from build123d import *

# Parameters (mm, degrees)
F0_R     = 26
F0_R_2   = 22.5
F0_R_3   = 15.5
F0_R_4   = 12.5
F1_DEPTH = 15
F3_R     = 5
F4_DEPTH = 11


with BuildPart() as f1:
    # F0 (on Front) → F1 (new body)
    with BuildSketch(Plane.XZ):
        Circle(F0_R)
        Circle(F0_R_2, mode=Mode.SUBTRACT)
        Circle(F0_R_3)
        Circle(F0_R_4, mode=Mode.SUBTRACT)
    extrude(amount=F1_DEPTH)

    # F3 (on offset) → F4 (join)
    with BuildSketch(Plane.XZ.offset(2)):
        with Locations((0, 19)):
            Circle(F3_R)
        with Locations((11.16792, 15.371323)):
            Circle(F3_R)
        with Locations((18.070074, 5.871323)):
            Circle(F3_R)
        with Locations((18.070074, -5.871323)):
            Circle(F3_R)
        with Locations((11.16792, -15.371323)):
            Circle(F3_R)
        with Locations((0, -19)):
            Circle(F3_R)
        with Locations((-11.16792, -15.371323)):
            Circle(F3_R)
        with Locations((-18.070074, -5.871323)):
            Circle(F3_R)
        with Locations((-18.070074, 5.871323)):
            Circle(F3_R)
        with Locations((-11.16792, 15.371323)):
            Circle(F3_R)
    extrude(amount=F4_DEPTH)


solid = f1.part
Build history of the part. All positions in model axes, mm. A direction names the side the tool comes from. Round coordinates to 2 decimals unless told otherwise and drop trailing zeros. Write each loop counter-clockwise with the first axis right and the second up, starting at its lowest first coordinate (ties: lowest second). Pieces come first, ordered by that corner, then holes. Notation, with made-up numbers: M 2.25,32 L 22.25,32 A26 cw 22.25,60 Z; hole C 68.5,-13 d6. An arc over 180 degrees is marked long. Answer in a Markdown table with one row per item.
1. Saw through at A-A (x = 0). List the corners of the cut face in (y, z), and give its area (3 significant figures).
Geometry check:
| item | result |
|---|---|
| outline | M -15,-26 L 0,-26 L 0,-22.5 L -2,-22.5 L -2,-15.5 L 0,-15.5 L 0,-12.5 L -15,-12.5 L -15,-15.5 L -13,-15.5 L -13,-22.5 L -15,-22.5 Z; M -15,12.5 L 0,12.5 L 0,15.5 L -2,15.5 L -2,22.5 L 0,22.5 L 0,26 L -15,26 L -15,22.5 L -13,22.5 L -13,15.5 L -15,15.5 Z |
| area | 349 mm2 |
2. Mould opens along Z. For faces 1 (the face through (-16.033, -7.423, 10.438)), 2 (the face through (-6.836, -7.423, 17.868)) say: +Z half, -Z half, draft (parallel to the pull), parting line (faces both ways), or undercut.
Geometry check:
| item | result |
|---|---|
| face 1 | undercut |
| face 2 | undercut |
3. Saw through at C-C (z = 19.5). List the corners of the cut face in (x, y).
Geometry check:
| item | result |
|---|---|
| outline | M -17.2,-15 L -11.22,-15 L -11.22,-13 L -8.35,-13 L -8.35,-2 L -11.22,-2 L -11.22,0 L -17.2,0 Z; M -4.97,-13 L 4.97,-13 L 4.97,-2 L -4.97,-2 Z; M 8.35,-13 L 11.22,-13 L 11.22,-15 L 17.2,-15 L 17.2,0 L 11.22,0 L 11.22,-2 L 8.35,-2 Z |
4. Probe L1, parallel to Z at x = 19, y = -3.25; L2, parallel to Y at x = 17.5, z = -1.5; L3, parallel to Z at x = 8.5, y = -6.25. List the from-to ranges inside material, lowest first. Write a range as [from, to].
Geometry check:
| item | result |
|---|---|
| L1 | [-17.75, -12.05], [-10.78, -0.96], [0.96, 10.78], [12.05, 17.75] |
| L2 | [-13, -2] |
| L3 | [-24.57, -20.83], [-19.6, -9.17], [9.17, 19.6], [20.83, 24.57] |
5. Flat gauge pins, fed straight in: P1, Ø1, axis at y = -12.5, z = -4.5, coming from the +X side; P2, Ø4.5, axis at x = -18.5, z = -4, coming from the +Y side; P3, Ø6, axis at x = 1.5, z = -18.5, coming from the -Y side. Where does each tip first touch, or does it go through?
Geometry check:
| item | result |
|---|---|
| P1 | x = 25.69 |
| P2 | y = -2 |
| P3 | y = -13 |
6. Which spindle directions (+Z, -Z, +X, -X, +Y, -Y) get a long thin tool onto all of the face, cutting with end or side? Do faces 3 (the face through (-18, -2, 6)), 4 (the face through (11, -13, -15)). Say none if no direction does.
Geometry check:
| item | result |
|---|---|
| face 3 | +Y |
| face 4 | -Y |
7. Saw through at B-B (z = 0). List the corners of the cut face in (x, y), and give its area (3 significant figures).
Geometry check:
| item | result |
|---|---|
| outline | M -26,-15 L -22.5,-15 L -22.5,0 L -26,0 Z; M -15.5,-15 L -12.5,-15 L -12.5,0 L -15.5,0 Z; M 12.5,-15 L 15.5,-15 L 15.5,0 L 12.5,0 Z; M 22.5,-15 L 26,-15 L 26,0 L 22.5,0 Z |
| area | 195 mm2 |
8. Saw through at D-D (x = 18). List the corners of the cut face in (y, z).
Geometry check:
| item | result |
|---|---|
| outline | M -15,-18.76 L 0,-18.76 L 0,-13.5 L -15,-13.5 Z; M -15,13.5 L 0,13.5 L 0,18.76 L -15,18.76 Z; M -13,-10.87 L -2,-10.87 L -2,-0.87 L -13,-0.87 Z; M -13,0.87 L -2,0.87 L -2,10.87 L -13,10.87 Z |
